from build123d import *

# Parameters (mm, degrees)
F0_W     = 115.1548996568
F0_H     = 142.901070416
F1_DEPTH = 7.62
F2_R     = 5.08
F3_W     = 5.0534754992
F3_H     = 43.796794489
F3_R     = 2.9202239124
F4_DEPTH = 7.62


# Not quite as in the source:
# - a feature names something its author has since deleted; it is built from what else it names


with BuildPart() as f1:
    # F0 (on Top) → F1 (new body)
    with BuildSketch(Plane.XY):
        with Locations((-0.3047175705, -0.2807490528)):
            Rectangle(F0_W, F0_H)
    extrude(amount=F1_DEPTH)

    # F2
    f2_edges = [f1.edges().sort_by_distance(p)[0] for p in [
        (-57.882167, -71.731284, 3.81),
        (-57.882167, 71.169786, 3.81),
        (57.272732, -71.731284, 3.81),
        (57.272732, 71.169786, 3.81),
    ]]
    fillet(f2_edges, radius=F2_R)

    # F3 (on face) + F0 (on Top) → F4 (cut)
    with BuildSketch(Plane.XY.offset(7.62)):
        with Locations((-50.8155077696, 0.4211226478)):
            Rectangle(F3_W, F3_H)
        with Locations((17.1256698668, 59.0975955129)):
            Circle(F3_R)
        with Locations((50.8155077696, 0.4211226478)):
            Rectangle(F3_W, F3_H)
        with Locations((-17.1256698668, 59.0975955129)):
            Circle(F3_R)
        with Locations((-17.1256698668, -59.0975955129)):
            Circle(F3_R)
        with Locations((17.1256698668, -59.0975955129)):
            Circle(F3_R)
    with BuildSketch(Plane.XY):
        with Locations((-0.3047175705, -0.2807490528)):
            Rectangle(F0_W, F0_H)
    extrude(amount=-F4_DEPTH, mode=Mode.SUBTRACT)


solid = f1.part
Can you work these out from the model? Positions are in its coordinate system, mm. A direction names the side the tool comes from. Give positions to 0.01 mm unless a question says otherwise; leave off trailing zeros. Loops run counter-clockwise (first coordinate to the right, second up) from the corner with the lowest first, then second, coordinate; pieces in that order, holes last. Notation, with made-up numbers: M 77.25,-15 L 133.25,-15 A13 ccw 133.25,10 Z; hole C 59,50.25 d5. An arc over 180 degrees is marked long. One line per item, written item: value.
1) Imagine slicing it at B-B on x = -16. Write out the boundary of the cut face in (y, z).
Geometry check:
outline: M -71.73,0 L -61.79,0 L -61.79,7.62 L -71.73,7.62 Z; M -56.4,0 L 56.4,0 L 56.4,7.62 L -56.4,7.62 Z; M 61.79,0 L 71.17,0 L 71.17,7.62 L 61.79,7.62 Z
2) Thinking about a two-plate mould opening in X: for faces 1 (the face through (51, 22.32, 4)), 2 (the face through (-51, -21.477, 4)), 3 (the face through (57.273, -1, 4)), 4 (the face through (-1, 1, 7.62)), which applies, +X half, -X half, draft (parallel to the pull), parting line (faces both ways), or undercut?
Geometry check:
face 1: undercut
face 2: undercut
face 3: +X half
face 4: draft
3) Imagine slicing it at C-C on z = 3.5. Write out the boundary of the cut face in (x, y), and give its area (3 significant figures).
Geometry check:
outline: M -57.88,-66.65 A5.08 ccw -52.8,-71.73 L 52.19,-71.73 A5.08 ccw 57.27,-66.65 L 57.27,66.09 A5.08 ccw 52.19,71.17 L -52.8,71.17 A5.08 ccw -57.88,66.09 Z; hole M -53.34,-21.48 L -48.29,-21.48 L -48.29,22.32 L -53.34,22.32 Z; hole C -17.13,-59.1 d5.84; hole C -17.13,59.1 d5.84; hole C 17.13,-59.1 d5.84; hole C 17.13,59.1 d5.84; hole M 48.29,-21.48 L 53.34,-21.48 L 53.34,22.32 L 48.29,22.32 Z
area: 15,900 mm²
4) On a 3-axis mill with a long thin cutter (end or side, diameter ignored), from which of +Z, -Z, +X, -X, +Y, -Y can I reach the whole of each face in a straight line? I mean faces 5 (the face through (-1, 1, 0)), 6 (the face through (53.342, 0, 4)). Say none if no direction works.
Geometry check:
face 5: -Z, +X, -X, +Y, -Y
face 6: +Z, -Z
5) Please list where these lines run through material, in increasing order: line 1 (X direction, y = -10, z = 0.75); line 2 (Y direction, x = 16, z = 4.5); line 3 (X direction, y = -60, z = 2.75).
Geometry check:
line 1: x = -57.88 to -53.34, -48.29 to 48.29, 53.34 to 57.27
line 2: y = -71.73 to -61.79, -56.4 to 56.4, 61.79 to 71.17
line 3: x = -57.88 to -19.9, -14.35 to 14.35, 19.9 to 57.27
6) Imagine slicing it at A-A on y = 11. Write out the boundary of the cut face in (x, z), and give its area (3 significant figures).
Geometry check:
outline: M -57.88,0 L -53.34,0 L -53.34,7.62 L -57.88,7.62 Z; M -48.29,0 L 48.29,0 L 48.29,7.62 L -48.29,7.62 Z; M 53.34,0 L 57.27,0 L 57.27,7.62 L 53.34,7.62 Z
area: 800 mm²
